from build123d import *

# Parameters (mm, degrees)
F0_W     = 203.2
F0_H     = 127
F1_DEPTH = 127
F3_DEPTH = 76.2
F4_SIZE2 = 101.6
F4_SIZE  = 76.2
F5_R     = 5.08
F6_R     = 15.24
F7_DEPTH = 50.8
F8_R     = 15.24
F9_DEPTH = 127


with BuildPart() as f1:
    # F0 (on Front) → F1 (new body)
    with BuildSketch(Plane.XZ):
        with Locations((-4.2091682553, -6.2115366554)):
            Rectangle(F0_W, F0_H)
    extrude(amount=F1_DEPTH)

    # F2 (on face) → F3 (cut)
    with BuildSketch(Plane.XZ.offset(127)):
        Polygon((97.3908317447, 57.2884633446), (-4.2091682553, 57.2884633446), (-4.2091682553, -6.2115366554), (-42.3091682553, -6.2115366554), (-42.3091682553, -69.7115366554), (97.3908317447, -69.7115366554), align=None)
    extrude(amount=-F3_DEPTH, mode=Mode.SUBTRACT)

    # F4
    f4_edges = [f1.edges().sort_by_distance(p)[0] for p in [
        (97.390832, -25.4, 57.288463),
    ]]
    f4_side = f1.faces().sort_by_distance((-25.980597, -52.614286, 57.288463))[0]
    chamfer(f4_edges, length=F4_SIZE, length2=F4_SIZE2, reference=f4_side)

    # F5
    f5_edges = [f1.edges().sort_by_distance(p)[0] for p in [
        (-55.009168, -127, 57.288463),
        (-4.209168, -88.9, 57.288463),
        (8.490832, -50.8, 57.288463),
        (21.190832, -25.4, 57.288463),
        (-4.209168, -127, 25.538463),
        (-23.259168, -127, -6.211537),
        (-42.309168, -127, -37.961537),
        (-74.059168, -127, -69.711537),
        (-105.809168, -127, -6.211537),
        (-42.309168, -88.9, -69.711537),
        (27.540832, -50.8, -69.711537),
        (97.390832, -25.4, -69.711537),
    ]]
    fillet(f5_edges, radius=F5_R)

    # F6 (on face) → F7 (cut)
    with BuildSketch(Plane.XZ.offset(50.8)):
        with Locations((8.4908317447, -20.9435366554)):
            Circle(F6_R)
    extrude(amount=-F7_DEPTH, mode=Mode.SUBTRACT)

    # F8 (on face) → F9 (cut, through all)
    with BuildSketch(Plane.XY.offset(57.2884633446)):
        with Locations((-85.3469744325, -90.6746312976)):
            Circle(F8_R)
    extrude(amount=-F9_DEPTH, mode=Mode.SUBTRACT)


solid = f1.part
Input: part model. Units: mm. Frame: model coordinates. A direction names the side the tool comes from. Give positions to 0.01 mm unless a question says otherwise; leave off trailing zeros. Write each loop counter-clockwise with the first axis right and the second up, starting at its lowest first coordinate (ties: lowest second). Pieces come first, ordered by that corner, then holes. Notation, with made-up numbers: M 22,30.5 L 67,30.5 A12 cw 67,53.5 Z; hole C 13.5,-0.75 d11. An arc over 180 degrees is marked long. Use one line per item in the form item = value.
1. Reachability of faces 4 (the face through (7.62, -49.27, 55.84)), 5 (the face through (-43.837, -83.287, -68.263)), 6 (the face through (95.942, -25.756, -68.184)) from +Z, -Z, +X, -X, +Y, -Y: full face, straight path, thin tool, end or side. Return the list, or none.
Outcome:
face_4 = +Z, +X, -Y
face_5 = -Z, +X, -Y
face_6 = -Z, +X, +Y, -Y
2. Cut plane D-D on z = 10. Return loops of the section in (x, y), and give its area (3 significant figures).
Outcome:
outline = M -105.81,-121.92 A5.08 ccw -100.73,-127 L -9.29,-127 A5.08 ccw -4.21,-121.92 L -4.21,-50.8 L 56.66,-50.8 L 56.66,0 L -105.81,0 Z; hole C -85.35,-90.67 d30.48
area = 15,300 mm²
3. Cut plane C-C on x = -33. Return loops of the section in (y, z).
Outcome:
outline = M -127,-1.13 A5.08 ccw -121.92,-6.21 L -50.8,-6.21 L -50.8,-64.63 A5.08 ccw -45.72,-69.71 L 0,-69.71 L 0,57.29 L -121.92,57.29 A5.08 ccw -127,52.21 Z
4. Cut plane A-A on z = -17.5. Return loops of the section in (x, y).
Outcome:
outline = M -105.81,-121.92 A5.08 ccw -100.73,-127 L -47.39,-127 A5.08 ccw -42.31,-121.92 L -42.31,-50.8 L -6.36,-50.8 L -6.36,0 L -105.81,0 Z; M 23.34,-50.8 L 77.28,-50.8 L 77.28,0 L 23.34,0 Z; hole C -85.35,-90.67 d30.48
5. Ray query, L1, parallel to X at y = -36, z = -29.5; L2, parallel to Z at x = -23.5, y = -76.5; L3, parallel to X at y = -79.5, z = 0.5. Return the intervals inside material, ascending.
Outcome:
L1 = -105.81 to -4.12, 21.1 to 86.28
L2 = -6.21 to 57.29
L3 = -105.81 to -95.71, -74.98 to -4.21
6. First-contact query: P1, Ø18.5, axis at x = 8.49, z = -20.94, coming from the +Y side; P2, Ø17.5, axis at y = -81.5, z = -29.5, coming from the +X side; P3, Ø6, axis at y = -65.5, z = -4.5, coming from the +X side; P4, Ø6, axis at y = -42.5, z = 30, coming from the +X side. Flat tips, straight axial feed; report the tip coordinate or a pass-through.
Outcome:
P1 = through
P2 = -42.31
P3 = -4.21
P4 = 43.91
7. Mould query, pull axis Y, two halves, no side actions, for faces 1 (the face through (-87.331, -75.564, -5.323)), 2 (the face through (-4.209, -87, 23)), 3 (the face through (-5.737, -125.551, 22.59)). Classes: released by +Y, released by -Y, zero draft, split by the parting line, or undercut.
Outcome:
face_1 = undercut
face_2 = zero draft
face_3 = released by -Y
8. Cut plane B-B on y = -95.5. Return loops of the section in (x, z), and give its area (3 significant figures).
Outcome:
outline = M -105.81,-69.71 L -99.8,-69.71 L -99.8,57.29 L -105.81,57.29 Z; M -70.89,-69.71 L -47.39,-69.71 A5.08 ccw -42.31,-64.63 L -42.31,-6.21 L -4.21,-6.21 L -4.21,52.21 A5.08 ccw -9.29,57.29 L -70.89,57.29 Z
area = 6,800 mm²
